Study the drawing (mm; zero at the part's minimum x, y, z) and answer. A direction names the side the tool comes from. Round coordinates to 2 decimals unless told otherwise and drop trailing zeros. Loops run counter-clockwise (first coordinate to the right, second up) from the corner with the lowest first, then second, coordinate; pieces in that order, holes last. Notation, with made-up numbers: (75.5, 5) - (132.5, 5) arc R21 ccw to (132.5, 26) - close; hole circle Ø4 at (72.5, -11.75). An arc over 180 degrees is marked (long way). One line per item, written item: value.
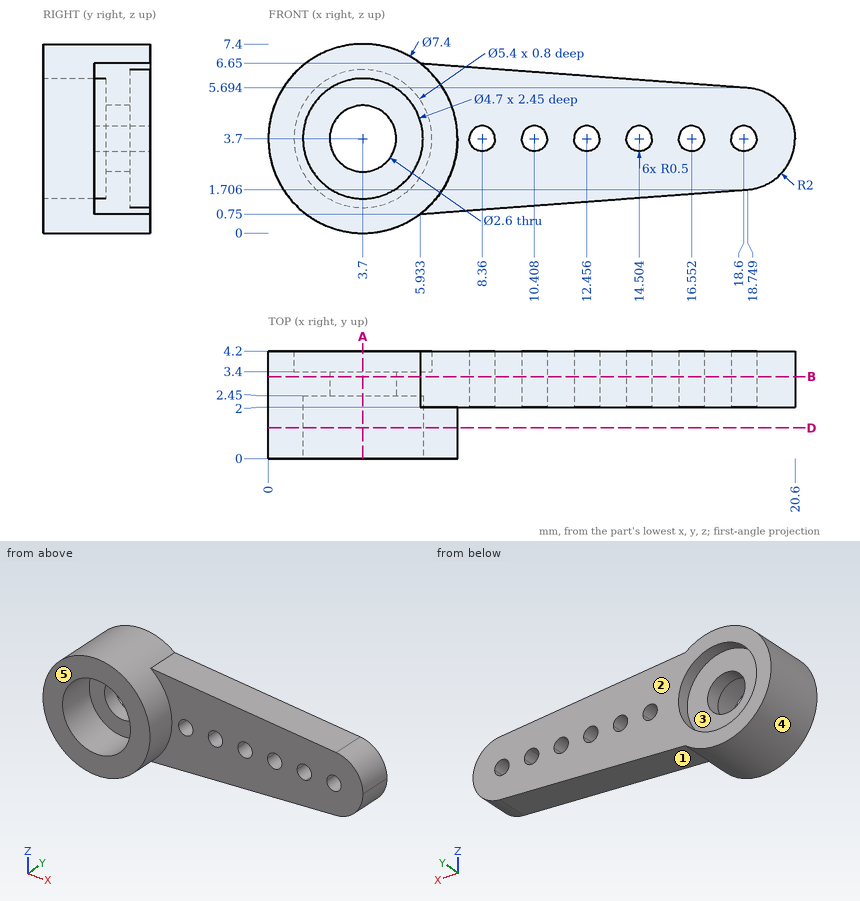
1) Each of these flat-tipped pins is pushed along its axis until it touches: pin 1 Ø1.8 at (x, z) = (12.5, 2.5) entering from -Y; pin 2 Ø3 at (x, z) = (3.7, 3.7) entering from +Y. Where does it stop, or does it pass through?
Final values:
pin 1: y = 2
pin 2: y = 3.4
2) For the marked faces 4 and 5, determine the directions among +Z, -Z, +X, -X, +Y, -Y from which every point of the face is accessible in a straight line to the end or side of a thin tool.
Final values:
face 4: -Y
face 5: +Z, -Z, +X, -X, -Y
3) A cutting plane is placed at B-B on y = 3.2. Give the number of separate pieces and of enclosed holes in the cut face.
Final values:
separate pieces: 1
enclosed holes: 7
4) For a pull along Z with two mould halves and no side action, classify the marked faces 1, 2 and 3 as released by +Z, released by -Z, zero draft, split by the parting line, or undercut.
Final values:
face 1: released by -Z
face 2: zero draft
face 3: undercut
5) Consider L1, parallel to X at y = 1.8, z = 3.7; L2, parallel to Y at x = 14.25, z = 1.5; L3, parallel to X at y = 0.5, z = 4.75. Determine where each line is inside the solid, lowest interval first.
Final values:
L1: 0 to 1.35, 6.05 to 7.4
L2: 2 to 4.2
L3: 0.15 to 1.6, 5.8 to 7.25
6) A cutting plane is placed at D-D on y = 1.2. Give the vertices of the cut face in (x, z).
Final values:
outline: circle Ø7.4 at (3.7, 3.7); hole circle Ø4.7 at (3.7, 3.7)
7) A cutting plane is placed at A-A on x = 3.7. Give the vertices of the cut face in (y, z).
Final values:
outline: (0, 0) - (4.2, 0) - (4.2, 1) - (3.4, 1) - (3.4, 2.4) - (2.45, 2.4) - (2.45, 1.35) - (0, 1.35) - close; (0, 6.05) - (2.45, 6.05) - (2.45, 5) - (3.4, 5) - (3.4, 6.4) - (4.2, 6.4) - (4.2, 7.4) - (0, 7.4) - close
